Solid Edge part; units mm, degrees
sketch "Sketch1" plane through (0, 0, 0) normal (0, 0, 1) x (1, 0, 0)
  line L0 (-110, -90) -> (110, -90)
  line L1 (110, -90) -> (110, 90)
  line L2 (110, 90) -> (-110, 90)
  line L3 (-110, 90) -> (-110, -90)
  circle A0 centre (-86, -66) radius 3.25
  circle A1 centre (-86, 66) radius 3.25
  circle A2 centre (86, -66) radius 3.25
  circle A3 centre (86, 66) radius 3.25
extrude "Protrusion1" add sketch "Sketch1" along normal blind 4
sketch "Sketch2" plane through (0, 0, 4) normal (0, 0, 1) x (1, 0, 0)
  line L0 (-110, -90) -> (110, -90)
  line L1 (110, -90) -> (110, 90)
  line L2 (110, 90) -> (-110, 90)
  line L3 (-110, 90) -> (-110, -90)
  line L4 (-107, -87) -> (107, -87)
  line L5 (107, -87) -> (107, 87)
  line L6 (107, 87) -> (-107, 87)
  line L7 (-107, 87) -> (-107, -87)
extrude "ExtrudedProtrusion_2" add sketch "Sketch2" along normal blind 88
sketch "Sketch3" plane through (0, 0, 4) normal (0, 0, 1) x (1, 0, 0)
  circle A0 centre (-102, -82) radius 7
extrude "ExtrudedProtrusion_3" add sketch "Sketch3" along normal blind 88
sketch "Sketch4" plane through (0, 0, 4) normal (0, 0, 1) x (1, 0, 0)
  circle A0 centre (-102, 82) radius 7
extrude "ExtrudedProtrusion_4" add sketch "Sketch4" along normal blind 88
sketch "Sketch5" plane through (0, 0, 4) normal (0, 0, 1) x (1, 0, 0)
  circle A0 centre (102, -82) radius 7
extrude "ExtrudedProtrusion_5" add sketch "Sketch5" along normal blind 88
sketch "Sketch6" plane through (0, 0, 4) normal (0, 0, 1) x (1, 0, 0)
  circle A0 centre (102, 82) radius 7
extrude "ExtrudedProtrusion_6" add sketch "Sketch6" along normal blind 88
sketch "Sketch7" plane through (0, 0, 4) normal (0, 0, 1) x (1, 0, 0)
  circle A0 centre (0, -82) radius 7
extrude "ExtrudedProtrusion_7" add sketch "Sketch7" along normal blind 88
sketch "Sketch8" plane through (0, 0, 4) normal (0, 0, 1) x (1, 0, 0)
  circle A0 centre (0, 82) radius 7
extrude "ExtrudedProtrusion_8" add sketch "Sketch8" along normal blind 88
sketch "Sketch9" plane through (0, 0, 84) normal (0, 0, 1) x (1, 0, 0)
  circle A0 centre (-102, -82) radius 1.7
  circle A1 centre (-102, 82) radius 1.7
  circle A2 centre (102, -82) radius 1.7
  circle A3 centre (102, 82) radius 1.7
  circle A4 centre (0, -82) radius 1.7
  circle A5 centre (0, 82) radius 1.7
extrude "ExtrudedCutout_1" cut sketch "Sketch9" along normal blind 8
sketch "Sketch10" plane through (0, 0, 89.3) normal (0, 0, 1) x (1, 0, 0)
  line L0 (-98.6514, -82) -> (-100.3257, -79.1)
  line L1 (-100.3257, -79.1) -> (-103.6743, -79.1)
  line L2 (-103.6743, -79.1) -> (-105.3486, -82)
  line L3 (-105.3486, -82) -> (-103.6743, -84.9)
  line L4 (-103.6743, -84.9) -> (-100.3257, -84.9)
  line L5 (-100.3257, -84.9) -> (-98.6514, -82)
  line L6 (-98.6514, 82) -> (-100.3257, 84.9)
  line L7 (-100.3257, 84.9) -> (-103.6743, 84.9)
  line L8 (-103.6743, 84.9) -> (-105.3486, 82)
  line L9 (-105.3486, 82) -> (-103.6743, 79.1)
  line L10 (-103.6743, 79.1) -> (-100.3257, 79.1)
  line L11 (-100.3257, 79.1) -> (-98.6514, 82)
  line L12 (105.3486, -82) -> (103.6743, -79.1)
  line L13 (103.6743, -79.1) -> (100.3257, -79.1)
  line L14 (100.3257, -79.1) -> (98.6514, -82)
  line L15 (98.6514, -82) -> (100.3257, -84.9)
  line L16 (100.3257, -84.9) -> (103.6743, -84.9)
  line L17 (103.6743, -84.9) -> (105.3486, -82)
  line L18 (105.3486, 82) -> (103.6743, 84.9)
  line L19 (103.6743, 84.9) -> (100.3257, 84.9)
  line L20 (100.3257, 84.9) -> (98.6514, 82)
  line L21 (98.6514, 82) -> (100.3257, 79.1)
  line L22 (100.3257, 79.1) -> (103.6743, 79.1)
  line L23 (103.6743, 79.1) -> (105.3486, 82)
  line L24 (3.3486, -82) -> (1.6743, -79.1)
  line L25 (1.6743, -79.1) -> (-1.6743, -79.1)
  line L26 (-1.6743, -79.1) -> (-3.3486, -82)
  line L27 (-3.3486, -82) -> (-1.6743, -84.9)
  line L28 (-1.6743, -84.9) -> (1.6743, -84.9)
  line L29 (1.6743, -84.9) -> (3.3486, -82)
  line L30 (3.3486, 82) -> (1.6743, 84.9)
  line L31 (1.6743, 84.9) -> (-1.6743, 84.9)
  line L32 (-1.6743, 84.9) -> (-3.3486, 82)
  line L33 (-3.3486, 82) -> (-1.6743, 79.1)
  line L34 (-1.6743, 79.1) -> (1.6743, 79.1)
  line L35 (1.6743, 79.1) -> (3.3486, 82)
extrude "ExtrudedCutout_2" cut sketch "Sketch10" along normal blind 2.7
sketch "Sketch11" plane through (0, 0, 16) normal (0, 0, 1) x (1, 0, 0)
  line L0 (-91, -92) -> (-25, -92)
  line L1 (-25, -92) -> (-25, -84)
  line L2 (-25, -84) -> (-91, -84)
  line L3 (-91, -84) -> (-91, -92)
extrude "ExtrudedCutout_3" cut sketch "Sketch11" along normal blind 20
sketch "Sketch12" plane through (0, 0, 0) normal (0, 0, 1) x (1, 0, 0)
  circle A0 centre (17, -43) radius 1.7
  circle A1 centre (63, -43) radius 1.7
  circle A2 centre (17, 18) radius 1.7
  circle A3 centre (63, 18) radius 1.7
extrude "ExtrudedCutout_4" cut sketch "Sketch12" along normal blind 4
sketch "Sketch13" plane through (0, 0, 0) normal (0, 0, 1) x (1, 0, 0)
  circle A0 centre (-84, -70) radius 1.7
  circle A1 centre (-84, -44) radius 1.7
  circle A2 centre (-26, -70) radius 1.7
  circle A3 centre (-26, -44) radius 1.7
extrude "ExtrudedCutout_5" cut sketch "Sketch13" along normal blind 4
Could you check a few things on this model? Use its own coordinates, in mm. A direction names the side the tool comes from. Coordinates: 2 decimals unless noted, no trailing zeros. Order: outer loops, then holes, each group sorted by start corner. A loop starts at its lowest first (then second) coordinate and runs counter-clockwise, first axis right, second up. Notation, with made-up numbers: (20, 79) - (78, 79) arc R23 cw to (78, 111) - close; hole circle Ø6 at (77, -40). An arc over 180 degrees is marked (long way). Answer in a Markdown table with one row per item. Add a question column.
(1) If we section it at C-C, the plane y = 50: Please give me the cut outline in (x, z), then the cut area to 3 significant figures.
(2) Will these pins go through, and if not, where does the flat tip stop? pin 1 (10.5 mm diameter, centred on x = 86, y = 66, fed in from +Z); pin 2 (2.5 mm diameter, centred on x = -102, y = 82.5, fed in from +Z).
(3) On a 3-axis mill with a long thin cutter (end or side, diameter ignored), from which of +Z, -Z, +X, -X, +Y, -Y can I reach the whole of each face in a straight line? I mean faces 1 (the face through (-107, 1, 47)), 2 (the face through (83.605, 63.803, 1.972)). Say none if no direction works.
(4) I need wall thicknesses on L1, parallel to Y at x = 0, z = 86.3; L2, parallel to X at y = 82, z = 86.65; L3, parallel to Y at x = 63, z = 2. Which ranges of each line are inside material? Lowest first, please.
(5) If we section it at B-B, the plane x = -37.5: Please give me the cut outline in (y, z).
(6) If we mould it in two halves opening along Y, with no side actions, what happens to faces 3 (the face through (-2, -90, 45)), 4 (the face through (-1, 87, 92)), 5 (the face through (0, 75, 47))? For each: released by +Y, released by -Y, zero draft, split by the parting line, or undercut.
Results are:
| question | item | result |
|---|---|---|
| 1 | outline | (-110, 0) - (110, 0) - (110, 92) - (107, 92) - (107, 4) - (-107, 4) - (-107, 92) - (-110, 92) - close |
| 1 | area | 1,410 mm2 |
| 2 | pin 1 | stops at z = 4 |
| 2 | pin 2 | stops at z = 89.3 |
| 3 | face 1 | +Z |
| 3 | face 2 | +Z, -Z |
| 4 | L1 | y = -90 to -83.7, -80.3 to -75, 75 to 80.3, 83.7 to 90 |
| 4 | L2 | x = -110 to -103.7, -100.3 to -95, -7 to -1.7, 1.7 to 7, 95 to 100.3, 103.7 to 110 |
| 4 | L3 | y = -90 to -44.7, -41.3 to 16.3, 19.7 to 90 |
| 5 | outline | (-90, 0) - (90, 0) - (90, 92) - (87, 92) - (87, 4) - (-87, 4) - (-87, 16) - (-90, 16) - close; (-90, 36) - (-87, 36) - (-87, 92) - (-90, 92) - close |
| 6 | face 3 | released by -Y |
| 6 | face 4 | zero draft |
| 6 | face 5 | undercut |
